from build123d import *

# Parameters (mm, degrees)
F0_R     = 1.89865
F1_DEPTH = 3.175


with BuildPart() as f1:
    # F0 (on Front) → F1 (new body)
    with BuildSketch(Plane.XZ):
        with BuildLine():
            Line((200.025, 95.25), (-200.025, 95.25))
            ThreePointArc((-200.025, 95.25), (-202.2700640303, 94.3200640303), (-203.2, 92.075))
            Line((-203.2, 92.075), (-203.2, -92.075))
            ThreePointArc((-203.2, -92.075), (-202.2700640303, -94.3200640303), (-200.025, -95.25))
            Line((-200.025, -95.25), (200.025, -95.25))
            ThreePointArc((200.025, -95.25), (202.2700640303, -94.3200640303), (203.2, -92.075))
            Line((203.2, -92.075), (203.2, 92.075))
            ThreePointArc((203.2, 92.075), (202.2700640303, 94.3200640303), (200.025, 95.25))
        make_face()
        with Locations((-152.4, -82.55)):
            Circle(F0_R, mode=Mode.SUBTRACT)
        with Locations((-101.6, -82.55)):
            Circle(F0_R, mode=Mode.SUBTRACT)
        with Locations((-149.6, -63.5)):
            Circle(F0_R, mode=Mode.SUBTRACT)
        with Locations((-50.8, -82.55)):
            Circle(F0_R, mode=Mode.SUBTRACT)
        with Locations((0, -82.55)):
            Circle(F0_R, mode=Mode.SUBTRACT)
        with Locations((-85.6, -63.5)):
            Circle(F0_R, mode=Mode.SUBTRACT)
        with Locations((-32, -63.5)):
            Circle(F0_R, mode=Mode.SUBTRACT)
        with BuildLine():
            ThreePointArc((-189.1, 1.9), (-188.1700640303, 4.1450640303), (-185.925, 5.075))
            Line((-185.925, 5.075), (-166.875, 5.075))
            ThreePointArc((-166.875, 5.075), (-164.6299359697, 4.1450640303), (-163.7, 1.9))
            Line((-163.7, 1.9), (-163.7, -48.9))
            ThreePointArc((-163.7, -48.9), (-164.6299359697, -51.1450640303), (-166.875, -52.075))
            Line((-166.875, -52.075), (-185.925, -52.075))
            ThreePointArc((-185.925, -52.075), (-188.1700640303, -51.1450640303), (-189.1, -48.9))
            Line((-189.1, -48.9), (-189.1, 1.9))
        make_face(mode=Mode.SUBTRACT)
        with BuildLine():
            ThreePointArc((-71.5, 1.9), (-70.5700640303, 4.1450640303), (-68.325, 5.075))
            Line((-68.325, 5.075), (-49.275, 5.075))
            ThreePointArc((-49.275, 5.075), (-47.0299359697, 4.1450640303), (-46.1, 1.9))
            Line((-46.1, 1.9), (-46.1, -48.9))
            ThreePointArc((-46.1, -48.9), (-47.0299359697, -51.1450640303), (-49.275, -52.075))
            Line((-49.275, -52.075), (-68.325, -52.075))
            ThreePointArc((-68.325, -52.075), (-70.5700640303, -51.1450640303), (-71.5, -48.9))
            Line((-71.5, -48.9), (-71.5, 1.9))
        make_face(mode=Mode.SUBTRACT)
        with Locations((50.8, -82.55)):
            Circle(F0_R, mode=Mode.SUBTRACT)
        with Locations((101.6, -82.55)):
            Circle(F0_R, mode=Mode.SUBTRACT)
        with BuildLine():
            ThreePointArc((33.89865, -63.5), (32, -65.39865), (30.10135, -63.5))
            ThreePointArc((30.10135, -63.5), (32, -61.60135), (33.89865, -63.5))
        make_face(mode=Mode.SUBTRACT)
        with Locations((85.6, -55.5)):
            Circle(F0_R, mode=Mode.SUBTRACT)
        with Locations((152.4, -82.55)):
            Circle(F0_R, mode=Mode.SUBTRACT)
        with Locations((149.6, -55.5)):
            Circle(F0_R, mode=Mode.SUBTRACT)
        with BuildLine():
            ThreePointArc((46.1, 1.9), (47.0299359697, 4.1450640303), (49.275, 5.075))
            Line((49.275, 5.075), (68.325, 5.075))
            ThreePointArc((68.325, 5.075), (70.5700640303, 4.1450640303), (71.5, 1.9))
            Line((71.5, 1.9), (71.5, -48.9))
            ThreePointArc((71.5, -48.9), (70.5700640303, -51.1450640303), (68.325, -52.075))
            Line((68.325, -52.075), (49.275, -52.075))
            ThreePointArc((49.275, -52.075), (47.0299359697, -51.1450640303), (46.1, -48.9))
            Line((46.1, -48.9), (46.1, 1.9))
        make_face(mode=Mode.SUBTRACT)
        with BuildLine():
            ThreePointArc((164.6916105596, 1.7320367783), (165.6215465293, 3.9771008086), (167.8666105596, 4.9070367783))
            Line((167.8666105596, 4.9070367783), (186.9166105596, 4.9070367783))
            ThreePointArc((186.9166105596, 4.9070367783), (189.1616745898, 3.9771008086), (190.0916105596, 1.7320367783))
            Line((190.0916105596, 1.7320367783), (190.0916105596, -49.0679632217))
            ThreePointArc((190.0916105596, -49.0679632217), (189.1616745898, -51.3130272519), (186.9166105596, -52.2429632217))
            Line((186.9166105596, -52.2429632217), (167.8666105596, -52.2429632217))
            ThreePointArc((167.8666105596, -52.2429632217), (165.6215465293, -51.3130272519), (164.6916105596, -49.0679632217))
            Line((164.6916105596, -49.0679632217), (164.6916105596, 1.7320367783))
        make_face(mode=Mode.SUBTRACT)
        with Locations((-149.6, 16.5)):
            Circle(F0_R, mode=Mode.SUBTRACT)
        with Locations((-85.6, 16.5)):
            Circle(F0_R, mode=Mode.SUBTRACT)
        with Locations((-32, 16.5)):
            Circle(F0_R, mode=Mode.SUBTRACT)
        with Locations((32, 16.5)):
            Circle(F0_R, mode=Mode.SUBTRACT)
        with Locations((85.6, 8.5)):
            Circle(F0_R, mode=Mode.SUBTRACT)
        with Locations((149.6, 8.5)):
            Circle(F0_R, mode=Mode.SUBTRACT)
    extrude(amount=F1_DEPTH)


solid = f1.part
The listing builds one solid part. Answer for the finished solid, in the listing's coordinates (mm). Round coordinates to 2 decimals unless told otherwise and drop trailing zeros. Order: outer loops, then holes, each group sorted by start corner. A loop starts at its lowest first (then second) coordinate and runs counter-clockwise, first axis right, second up. Notation, with made-up numbers: (35, -4.75) - (45, -4.75) arc R25 ccw to (45, 7.25) - close; hole circle Ø5 at (86.25, 67.25). An arc over 180 degrees is marked (long way). Write item = value, one per line. Start each with the question number.
1) Given pin 1 (3 mm diameter, centred on x = 85.6, z = -55.5, fed in from -Y), flat-ended and moving along its own axis, determine where the tip first touches the part or whether it passes through.
2) Section A-A, the plane z = -43 is taken. Write down the section's boundary in (x, y) (3 decimals).
3) Straight lines are drawn through the part: L1, parallel to Z at x = -85.6, y = -2.45; L2, parallel to X at y = -1, z = -36; L3, parallel to Z at x = 149.6, y = -1.4. For each, find the intervals that lie inside material, in ascending order.
Results list:
q1.pin_1 = through
q2.outline = (-203.2, -3.175) - (-189.1, -3.175) - (-189.1, 0) - (-203.2, 0) - close; (-163.7, -3.175) - (-71.5, -3.175) - (-71.5, 0) - (-163.7, 0) - close; (-46.1, -3.175) - (46.1, -3.175) - (46.1, 0) - (-46.1, 0) - close; (71.5, -3.175) - (164.692, -3.175) - (164.692, 0) - (71.5, 0) - close; (190.092, -3.175) - (203.2, -3.175) - (203.2, 0) - (190.092, 0) - close
q3.L1 = -95.25 to -65.4, -61.6 to 14.6, 18.4 to 95.25
q3.L2 = -203.2 to -189.1, -163.7 to -71.5, -46.1 to 46.1, 71.5 to 164.69, 190.09 to 203.2
q3.L3 = -95.25 to -57.4, -53.6 to 6.6, 10.4 to 95.25
